from build123d import *

# Parameters (mm, degrees)
F0_R     = 1.5
F1_DEPTH = 4


with BuildPart() as f1:
    # F0 (on Front) → F1 (new body)
    with BuildSketch(Plane.XZ):
        Polygon((80, 15), (0, 15), (0, 5), (5, 0), (10, 5), (15, 0), (20, 5), (25, 0), (30, 5), (35, 0), (40, 5), (45, 0), (50, 5), (55, 0), (60, 5), (65, 0), (70, 5), (75, 0), (80, 5), align=None)
        with Locations((7.5, 7.5)):
            Circle(F0_R, mode=Mode.SUBTRACT)
    extrude(amount=F1_DEPTH)


solid = f1.part
Design review of the part built by this model. Coordinates are the model's own, in mm. A direction names the side the tool comes from. Coordinates: 2 decimals unless noted, no trailing zeros. Order: outer loops, then holes, each group sorted by start corner. A loop starts at its lowest first (then second) coordinate and runs counter-clockwise, first axis right, second up.
Item 1: Take a section at B-B, the plane y = -1.65. Write out the cut boundary in (x, z).
Item 2: For pin 1 Ø8 at (x, z) = (44.5, 5) entering from +Y, flat-tipped, find the tip position at first contact; note if it passes through.
Item 3: For line 1 (X direction, y = -1.75, z = 7); line 2 (X direction, y = -2.85, z = 8.75); line 3 (Z direction, x = 8, y = -2.9), list the stretches that pass through material, from the lowest coordinate up.
Item 4: The part is to be moulded in two halves that separate along X. For faces 3 (the flat face through (77, -2, 2)), 4 (the flat face through (67, -2, 2)), 5 (the flat face through (39, 0, 9)), say which applies: pulls with the +X half, pulls with the -X half, needs draft (parallel to the pull), parting line crosses it, or undercut.
Item 5: For faces 1 (the flat face through (41, -2, 15)), 2 (the flat face through (47, -2, 2)), list the 3-axis set-ups (+Z, -Z, +X, -X, +Y, -Y) from which the entire face can be reached by the end or side of a thin tool; tool diameter is ignored.
Item 6: Take a section at D-D, the plane x = 7.5. Write out the cut boundary in (y, z), then the cut area to 3 significant figures.
Item 7: Take a section at A-A, the plane z = 7.5. Write out the cut boundary in (x, y), then the cut area to 3 significant figures.
Item 8: Take a section at C-C, the plane z = 3.5. Count the separate pieces of the cut face and the enclosed holes in it, then the cut area to 3 significant figures.
The answers:
1. outline: (0, 5) - (5, 0) - (10, 5) - (15, 0) - (20, 5) - (25, 0) - (30, 5) - (35, 0) - (40, 5) - (45, 0) - (50, 5) - (55, 0) - (60, 5) - (65, 0) - (70, 5) - (75, 0) - (80, 5) - (80, 15) - (0, 15) - close; hole circle Ø3 at (7.5, 7.5)
2. pin 1: stops at y = 0
3. line 1: x = 0 to 6.09, 8.91 to 80
3. line 2: x = 0 to 6.67, 8.33 to 80
3. line 3: z = 3 to 6.09, 8.91 to 15
4. face 3: pulls with the +X half
4. face 4: undercut
4. face 5: needs draft
5. face 1: +Z, +X, -X, +Y, -Y
5. face 2: -Z, +Y, -Y
6. outline: (-4, 2.5) - (0, 2.5) - (0, 6) - (-4, 6) - close; (-4, 9) - (0, 9) - (0, 15) - (-4, 15) - close
6. area: 38.0 mm2
7. outline: (0, -4) - (6, -4) - (6, 0) - (0, 0) - close; (9, -4) - (80, -4) - (80, 0) - (9, 0) - close
7. area: 308 mm2
8. separate pieces: 8
8. enclosed holes: 0
8. area: 224 mm2
